```python
from build123d import *

# Parameters (mm, degrees)
F1_DEPTH = 75.438
F2_R     = 18.7791754174
F3_T     = -2.54
F5_D     = 6.35


# Not quite as in the source:
# - a shell that OpenCascade refuses in one call is made with other operations: the cavity is built on its own and cut out


with BuildPart() as f1:
    # F0 (on Top) → F1 (new body)
    with BuildSketch(Plane.XY):
        Polygon((0, 45.7287728786), (0, 0), (26.4172311872, 0), (49.5915971696, 45.7287728786), align=None)
    extrude(amount=F1_DEPTH)

    # F2
    f2_edges = [f1.edges().sort_by_distance(p)[0] for p in [
        (38.004414, 22.864386, 75.438),
    ]]
    fillet(f2_edges, radius=F2_R)

    # F3: a shell. OpenCascade refuses it in one call, so the cavity is built on its own and cut out:
    # the body offset inwards by the wall thickness, plus a prism from it out through each open face.
    f3_core = offset(f1.part, amount=F3_T, kind=Kind.INTERSECTION, mode=Mode.PRIVATE)
    f3_exits = [f3_core.faces().sort_by_distance(p)[0] for p in [
        (10.972623, 27.706391, 72.898),
    ]]
    add(f3_core, mode=Mode.SUBTRACT)
    extrude(f3_exits, amount=-F3_T, mode=Mode.SUBTRACT)

    # F5 (through all)
    with Locations(Plane(origin=(21.0190277096, -10.6519945775, 0), x_dir=(0.4520442786, 0.891995499, 0), z_dir=(0.891995499, -0.4520442786, 0))):
        with Locations((33.8537804782, 31.7050926387)):
            Hole(F5_D / 2)


solid = f1.part
```
Geometry: final body of the model. Coordinates: model frame, mm. A direction names the side the tool comes from. Coordinates: 2 decimals unless noted, no trailing zeros. Order: outer loops, then holes, each group sorted by start corner. A loop starts at its lowest first (then second) coordinate and runs counter-clockwise, first axis right, second up. Notation, with made-up numbers: (0.5, -24.5) - (43.5, -24.5) arc R20 cw to (43.5, -8.5) - close; hole circle Ø4 at (56, 25.5). An arc over 180 degrees is marked (long way). Return JSON: item names as keys, results as strings. Group by question number.
1. Material intervals for line 1 along Y through (x, z) = (24, 40.5); line 2 along X through (y, z) = (14, 24); line 3 along Z through (x, y) = (20, 29), sorted ascending. Write a range as [from, to].
2. Pin query (flat end, axial travel): pin 1 (20.5 mm diameter, centred on y = 22.5, z = 40, fed in from +X); pin 2 (10 mm diameter, centred on y = 21.5, z = 13, fed in from +X); pin 3 (4 mm diameter, centred on x = 15.5, y = 25, fed in from +Z). Return the tip coordinate at first contact, or that it passes through.
3. Cut plane B-B (z = 68). Output: boundary loops of the cut face in (x, y), plus the area to 3 significant figures.
4. Cut plane A-A (z = 25.5). Output: boundary loops of the cut face in (x, y), plus the area to 3 significant figures.
5. Pull-direction query (Y, two-part tool) for faces 1 (the face through (37.84, 22.54, 27.93)), 2 (the face through (0, 23, 37)), 3 (the face through (14, 2.54, 38)); classes: pulls with the +Y half, pulls with the -Y half, needs draft (parallel to the pull), parting line crosses it, or undercut.
6. Set-up query: faces 4 (the face through (24, 43.189, 38)), 5 (the face through (2.54, 23, 38)), 6 (the face through (2, 31, 75.438)). Return all of +Z, -Z, +X, -X, +Y, -Y with unobstructed straight access to the full face (end or side cutting, diameter ignored); none if empty.
Resolved:
{
 "1": {"line 1": "y = [0, 2.54], [43.19, 45.73]", "line 2": "x = [0, 2.54], [30.66, 33.51]", "line 3": "z = [0, 2.54]"},
 "2": {"pin 1": "stops at x = 43.01", "pin 2": "stops at x = 39.85", "pin 3": "stops at z = 2.54"},
 "3": {"outline": "(0, 0) - (22.14, 0) - (45.32, 45.73) - (0, 45.73) - close; hole (2.54, 2.54) - (19.68, 2.54) - (40.28, 43.19) - (2.54, 43.19) - close", "area": "427 mm²"},
 "4": {"outline": "(0, 0) - (26.42, 0) - (49.59, 45.73) - (0, 45.73) - close; hole (2.54, 2.54) - (24.86, 2.54) - (45.46, 43.19) - (2.54, 43.19) - close", "area": "412 mm²"},
 "5": {"face 1": "pulls with the -Y half", "face 2": "needs draft", "face 3": "undercut"},
 "6": {"face 4": "none", "face 5": "+Z", "face 6": "+Z, +X, -X, +Y, -Y"}
}
